Check sheet for the modelled part. Datum: model origin and axes. Units: mm. A direction names the side the tool comes from. Round coordinates to 2 decimals unless told otherwise and drop trailing zeros. Order: outer loops, then holes, each group sorted by start corner. A loop starts at its lowest first (then second) coordinate and runs counter-clockwise, first axis right, second up.
from build123d import *

# Parameters (mm, degrees)
BOSS_EXTRU_1_DEPTH      = 5.5
ESQUISSE3_R             = 2.5
ENL_V_MAT_EXTRU_1_DEPTH = 5.5
ESQUISSE4_R             = 9
BOSS_EXTRU_3_DEPTH      = 4.6
ESQUISSE2_R             = 35
BOSS_EXTRU_2_DEPTH      = 23.3
ESQUISSE5_R             = 16
BOSS_EXTRU_4_DEPTH      = 21


with BuildPart() as part:
    # Esquisse1 → Boss.-Extru.1 (new body)
    with BuildSketch(Plane.XY):
        with BuildLine():
            add(Edge.make_bspline(
                [(96.74, 35.14), (96.700966604, 46.914828886), (76.669243873, 62.532909125), (43.186721807, 70.453815297), (35, 70.14)],
                knots=[0, 0, 0, 0, 0.420118968, 1, 1, 1, 1], degree=3))
            add(Edge.make_bspline(
                [(35, 70.14), (29.89922146, 70.296066514), (19.629650744, 68.989823621), (9.641451794, 67.514202382), (5.51358225, 65.29011499)],
                knots=[0, 0, 0, 0, 0.536066819, 1, 1, 1, 1], degree=3))
            add(Edge.make_bspline(
                [(5.51358225, 65.29011499), (1.61130463, 61.662907457), (1.250702971, 49.999272028), (-0.535437112, 34.426866806), (0.654932347, 19.165653112), (2.922501297, 9.271234675), (5.092204, 5.66435325)],
                knots=[0, 0, 0, 0, 0.25720549, 0.505904817, 0.797009019, 1, 1, 1, 1], degree=3))
            add(Edge.make_bspline(
                [(96.74, 35.14), (95.57744451, 24.437841166), (74.678338114, 6.386866594), (40.041164519, -1.581693557), (14.123677955, 0.659923037), (5.092204, 5.66435325)],
                knots=[0, 0, 0, 0, 0.293375681, 0.712147859, 1, 1, 1, 1], degree=3))
        make_face()
    extrude(amount=BOSS_EXTRU_1_DEPTH)

    # Esquisse3 → Enlèv. mat.-Extru.1 (cut)
    with BuildSketch(Plane.XY.offset(5.5)):
        with Locations((7.5, 62.78)):
            Circle(ESQUISSE3_R)
        with Locations((7.5, 7.5)):
            Circle(ESQUISSE3_R)
        with Locations((77, 14.64)):
            Circle(ESQUISSE3_R)
        with Locations((77, 55.64)):
            Circle(ESQUISSE3_R)
    extrude(amount=-ENL_V_MAT_EXTRU_1_DEPTH, mode=Mode.SUBTRACT)

    # Esquisse4 → Boss.-Extru.3 (add)
    with BuildSketch(Plane.XY.offset(5.5)):
        with Locations((80.5, 35.14)):
            Circle(ESQUISSE4_R)
    extrude(amount=BOSS_EXTRU_3_DEPTH)

    # Esquisse2 → Boss.-Extru.2 (add)
    with BuildSketch(Plane.XY.offset(5.5)):
        with Locations(Location((35, 35.113142172, 0), (0, 0, 179.955291193))):
            Circle(ESQUISSE2_R)
    extrude(amount=BOSS_EXTRU_2_DEPTH)

    # Esquisse5 → Boss.-Extru.4 (add)
    with BuildSketch(Plane(origin=(0, 0, 0), x_dir=(-1, 0, 0), z_dir=(0, 0, -1))):
        with Locations(Location((-80.5, 35.14, 0), (0, 0, 190.060871127))):
            Circle(ESQUISSE5_R)
    extrude(amount=BOSS_EXTRU_4_DEPTH)


solid = part.part
1) Gauge pin test, flat ends, axial feed: pin 1 (1.5 mm diameter, centred on x = 18.5, z = 11, fed in from +Y); pin 2 (2 mm diameter, centred on x = 40, z = 17, fed in from +Y); pin 3 (8 mm diameter, centred on y = 51, z = -1.5, fed in from +X); pin 4 (4 mm diameter, centred on x = 7.5, y = 62.78, fed in from +Z). Record the tip position at first contact, or that the pin passes through.
2) Sectioned sample at C-C on z = -9. Record the cut outline in (x, y), and give its area (3 significant figures).
3) Draft check along X on faces 5 (the face through (8.65, 5.28, 2.79)), 6 (the face through (80, 35, -21)), 7 (the face through (64.64, 37.24, -10.35)). Enter one of: pulls with the +X half, pulls with the -X half, needs draft (parallel to the pull), parting line crosses it, or undercut.
4) Scan lines: line 1 (Y direction, x = 77, z = 3.6); line 2 (Z direction, x = 76, y = 37); line 3 (Z direction, x = 6.5, y = 52). Record each from-to range of solid material in increasing order.
5) Set-up check for faces 1 (the face through (80, 35, 10.1)), 2 (the face through (89.1, 37.8, 7.8)), 3 (the face through (35, 35, 28.8)), 4 (the face through (9, 10, 5.5)): record each of +Z, -Z, +X, -X, +Y, -Y from which the full face is reachable in a straight line by a thin tool's end or side.
6) Sectioned sample at A-A on z = 23. Record the cut outline in (x, y), and give its area (3 significant figures).
7) Sectioned sample at B-B on x = 7.5. Count the separate pieces of the cut face and the enclosed holes in it, and give its area (3 significant figures).
Values found:
1. pin 1: stops at y = 66.37
1. pin 2: stops at y = 69.88
1. pin 3: stops at x = 92.86
1. pin 4: passes through
2. outline: circle Ø32 at (80.5, 35.14)
2. area: 804 mm2
3. face 5: undercut
3. face 6: needs draft
3. face 7: parting line crosses it
4. line 1: y = 11.26 to 12.14, 17.14 to 53.14, 58.14 to 58.92
4. line 2: z = -21 to 10.1
4. line 3: z = 0 to 28.8
5. face 1: +Z, +X, +Y, -Y
5. face 2: +Z
5. face 3: +Z, +X, -X, +Y, -Y
5. face 4: +Z, -X, -Y
6. outline: circle Ø70 at (35, 35.11)
6. area: 3,850 mm2
7. separate pieces: 3
7. enclosed holes: 0
7. area: 1,290 mm2
